Geometry check sheet. Reference: the model listing, model coordinates, mm. A direction names the side the tool comes from. Round coordinates to 2 decimals unless told otherwise and drop trailing zeros. Order: outer loops, then holes, each group sorted by start corner. A loop starts at its lowest first (then second) coordinate and runs counter-clockwise, first axis right, second up. Notation, with made-up numbers: (-40, 87.25) -> (-1, 87.25) arc R15 cw to (-1, 93.25) -> close; hole circle Ø1 at (86.5, 80). An arc over 180 degrees is marked (long way). Use a Markdown table: item, result. Add a question column.
Item 1: Sectioned sample at C-C, the plane z = -279. Record the cut outline in (x, y).
Item 2: Material ranges on probe 1 along Z at (x, y) = (59, 0.9); probe 2 along Z at (x, y) = (119.5, 1.35); probe 3 along X at (y, z) = (1.7, -269), recorded low to high. Write a range as [from, to].
Item 3: Set-up check for faces 4 (the cylindrical face through (64.33, 1.52, -237.96)), 5 (the cylindrical face through (76.228, 1.521, -281.357)): record each of +Z, -Z, +X, -X, +Y, -Y from which the full face is reachable in a straight line by a thin tool's end or side.
Item 4: Mould release check, pull along X, two halves, no side actions. Record for faces 1 (the flat face through (140.858, 1.479, -246.973)), 2 (the flat face through (64, 3, -244)), 3 (the cylindrical face through (10.84, 1.52, -288.23)): pulls with the +X half, pulls with the -X half, needs draft (parallel to the pull), parting line crosses it, or undercut.
Item 5: Sectioned sample at A-A, the plane y = 0.55. Record the cut outline in (x, z).
Item 6: Sectioned sample at B-B, the plane x = 127. Record the cut outline in (y, z).
from build123d import *

# Parameters (mm, degrees)
BOSS_EXTRUDE1_DEPTH = 3
CUT_EXTRUDE1_DEPTH  = 3
FILLET1_R           = 10
FILLET2_R           = 3
BOSS_EXTRUDE2_DEPTH = 3
CUT_EXTRUDE2_DEPTH  = 3


with BuildPart() as part:
    # Sketch1 → Boss-Extrude1 (new body)
    with BuildSketch(Plane(origin=(0, 0, 0), x_dir=(1, 0, 0), z_dir=(0, 1, 0))):
        with BuildLine():
            Line((1.5, 297.496218463), (1.5, 271.496218463))
            ThreePointArc((1.5, 271.496218463), (70.269464473, 262.249211634), (134.449071126, 235.872622221))
            Line((134.449071126, 235.872622221), (147.449071126, 258.389282719))
            ThreePointArc((147.449071126, 258.389282719), (76.998665918, 287.362933321), (1.5, 297.496218463))
        make_face()
    extrude(amount=BOSS_EXTRUDE1_DEPTH)

    # Sketch3 → Cut-Extrude1 (cut)
    with BuildSketch(Plane(origin=(0, 3, 0), x_dir=(1, 0, 0), z_dir=(0, 1, 0))):
        with BuildLine():
            Line((7.5, 271.396751344), (129.203185143, 238.786481168))
            Line((129.203185143, 238.786481168), (136.70589842, 251.781561758))
            ThreePointArc((136.70589842, 251.781561758), (74.15175015, 276.738099028), (7.5, 286.402177897))
            Line((7.5, 286.402177897), (7.5, 271.396751344))
        make_face()
    extrude(amount=-CUT_EXTRUDE1_DEPTH, mode=Mode.SUBTRACT)

    # Fillet1
    fillet1_edges = [part.edges().sort_by_distance(p)[0] for p in [
        (7.5, 1.5, -286.402177897),
        (136.70589842, 1.5, -251.781561758),
    ]]
    fillet(fillet1_edges, radius=FILLET1_R)

    # Fillet2
    fillet2_edges = [part.edges().sort_by_distance(p)[0] for p in [
        (7.5, 1.5, -271.396751344),
        (129.203185143, 1.5, -238.786481168),
    ]]
    fillet(fillet2_edges, radius=FILLET2_R)

    # Sketch4 → Boss-Extrude2 (add)
    with BuildSketch(Plane(origin=(0, 3, 0), x_dir=(1, 0, 0), z_dir=(0, 1, 0))):
        with BuildLine():
            Line((129.252918703, 238.872622221), (130.736546702, 241.442341293))
            Line((130.736546702, 241.442341293), (134.449071126, 235.872622221))
            ThreePointArc((134.449071126, 235.872622221), (119.700341049, 223.942829747), (100.758430139, 224.967036005))
            ThreePointArc((100.758430139, 224.967036005), (63.798988345, 238.101065977), (25.224157857, 245.206383264))
            ThreePointArc((25.224157857, 245.206383264), (8.307878683, 253.79035008), (1.5, 271.496218463))
            Line((1.5, 271.496218463), (7.5, 274.46347446))
            Line((7.5, 274.46347446), (7.5, 271.496218463))
            ThreePointArc((7.5, 271.496218463), (12.762306102, 257.810061061), (25.838132399, 251.174886867))
            ThreePointArc((25.838132399, 251.174886867), (65.351902616, 243.896620934), (103.21096439, 230.44289902))
            ThreePointArc((103.21096439, 230.44289902), (117.852549236, 229.651215281), (129.252918703, 238.872622221))
        make_face()
    extrude(amount=-BOSS_EXTRUDE2_DEPTH)

    # Sketch5 → Cut-Extrude2 (cut)
    with BuildSketch(Plane(origin=(0, 3, 0), x_dir=(1, 0, 0), z_dir=(0, 1, 0))):
        with BuildLine():
            Line((131.477814314, 242.72625446), (133.824291098, 246.790471469))
            ThreePointArc((133.824291098, 246.790471469), (134.763656185, 254.918092038), (129.480348672, 261.165274172))
            ThreePointArc((129.480348672, 261.165274172), (75.445845375, 281.56772816), (18.449365845, 290.915936355))
            ThreePointArc((18.449365845, 290.915936355), (10.750296256, 288.147371682), (7.5, 280.638963253))
            Line((7.5, 280.638963253), (7.5, 275.946009685))
            Line((7.5, 275.946009685), (131.477814314, 242.72625446))
        make_face()
    extrude(amount=-CUT_EXTRUDE2_DEPTH, mode=Mode.SUBTRACT)


solid = part.part
Found:
| question | item | result |
|---|---|---|
| 1 | outline | (1.5, 0) -> (7.5, 0) -> (7.5, 3) -> (1.5, 3) -> close; (84.45, 0) -> (103.27, 0) -> (103.27, 3) -> (84.45, 3) -> close |
| 2 | probe 1 | z = [-291.59, -285.47], [-245.51, -239.34] |
| 2 | probe 2 | z = [-272.44, -265.88], [-230.26, -223.88] |
| 2 | probe 3 | x = [1.62, 7.65], [112.3, 127.06] |
| 3 | face 4 | +Z, -X, +Y, -Y |
| 3 | face 5 | +Y, -Y |
| 4 | face 1 | pulls with the +X half |
| 4 | face 2 | needs draft |
| 4 | face 3 | undercut |
| 5 | outline | (1.5, -297.5) arc R297.5 ccw to (147.45, -258.39) -> (134.45, -235.87) arc R26.43 ccw to (100.76, -224.97) arc R246.5 cw to (25.22, -245.21) arc R26.43 ccw to (1.5, -271.5) -> close; hole (7.5, -280.64) arc R10.3 ccw to (18.45, -290.92) arc R291.5 ccw to (129.48, -261.17) arc R10.3 ccw to (133.82, -246.79) -> (129.25, -238.87) arc R20.43 ccw to (103.21, -230.44) arc R252.5 cw to (25.84, -251.17) arc R20.43 ccw to (7.5, -271.5) -> close |
| 6 | outline | (0, -269.03) -> (3, -269.03) -> (3, -262.38) -> (0, -262.38) -> close; (0, -235.71) -> (3, -235.71) -> (3, -227.64) -> (0, -227.64) -> close |
